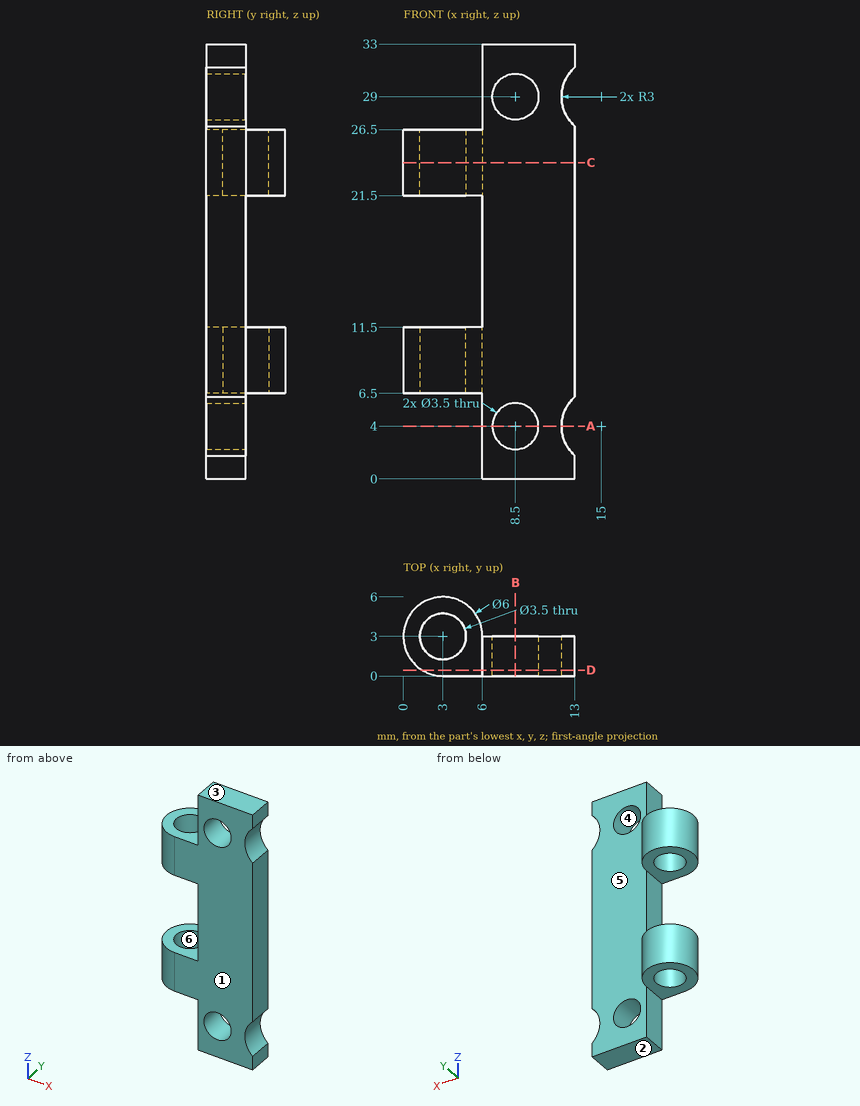
Geometry check sheet. Reference: drawing and pictorial views, mm from the part's lowest x, y, z. A direction names the side the tool comes from. Round coordinates to 2 decimals unless told otherwise and drop trailing zeros. Order: outer loops, then holes, each group sorted by start corner. A loop starts at its lowest first (then second) coordinate and runs counter-clockwise, first axis right, second up. Notation, with made-up numbers: M 26,3.25 L 81,3.25 A18 cw 81,8.25 Z; hole C 42.5,78.5 d7. An arc over 180 degrees is marked long. One line per item, written item: value. Start each with the question number.
1. Gauge pin test, flat ends, axial feed: P1, Ø1.5, axis at y = 1, z = 18.5, coming from the -X side; P2, Ø1.8, axis at x = 2.5, y = 4, coming from the +Z side; P3, Ø1.8, axis at x = 3, y = 2, coming from the -Z side. Record the tip position at first contact, or that the pin passes through.
2. Access from +Z, -Z, +X, -X, +Y, -Y to the whole of each face (thin tool, end or side, straight path). Record for the marked faces 5 and 6.
3. Scan lines: line 1 along Z through (x, y) = (8.5, 1.65); line 2 along Y through (x, z) = (3, 23.8); line 3 along X through (y, z) = (0.85, 29). Record each from-to range of solid material in increasing order.
4. Section check A-A on z = 4. Enter the section's corners in (x, y), and give its area (3 significant figures).
5. Section check B-B on x = 8.5. Enter the section's corners in (y, z), and give its area (3 significant figures).
6. Section check C-C on z = 24. Enter the section's corners in (x, y), and give its area (3 significant figures).
7. Release check for a two-part mould opening along Z. For the marked faces 1, 2, 3 and 4 record: released by +Z, released by -Z, zero draft, split by the parting line, or undercut.
8. Section check D-D on y = 0.45. Enter the section's corners in (x, z), and give its area (3 significant figures).
Results found:
1. P1: x = 6
1. P2: z = 26.5
1. P3: z = 6.5
2. face 5: +Z, -Z, +X, +Y
2. face 6: +Z, -Z
3. line 1: 0 to 2.25, 5.75 to 27.25, 30.75 to 33
3. line 2: 0 to 1.25, 4.75 to 6
3. line 3: 6 to 6.75, 10.25 to 12
4. outline: M 6,0 L 6.75,0 L 6.75,3 L 6,3 Z; M 10.25,0 L 12,0 L 12,3 L 10.25,3 Z
4. area: 7.50 mm^2
5. outline: M 0,0 L 3,0 L 3,2.25 L 0,2.25 Z; M 0,5.75 L 3,5.75 L 3,27.25 L 0,27.25 Z; M 0,30.75 L 3,30.75 L 3,33 L 0,33 Z
5. area: 78.0 mm^2
6. outline: M 3,0 L 13,0 L 13,3 L 6,3 A3 ccw long Z; hole C 3,3 d3.5
6. area: 41.6 mm^2
7. face 1: zero draft
7. face 2: released by -Z
7. face 3: released by +Z
7. face 4: undercut
8. outline: M 1.42,6.5 L 6,6.5 L 6,0 L 13,0 L 13,1.76 A3 cw 13,6.24 L 13,26.76 A3 cw 13,31.24 L 13,33 L 6,33 L 6,26.5 L 1.42,26.5 L 1.42,21.5 L 6,21.5 L 6,11.5 L 1.42,11.5 Z; hole C 8.5,4 d3.5; hole C 8.5,29 d3.5
8. area: 251 mm^2
